The listing builds one solid part. Answer for the finished solid, in the listing's coordinates (mm). Face numbers are marked on the shaded views. A direction names the side the tool comes from. Round coordinates to 2 decimals unless told otherwise and drop trailing zeros. Order: outer loops, then holes, each group sorted by start corner. A loop starts at its lowest first (then second) coordinate and runs counter-clockwise, first axis right, second up. Notation, with made-up numbers: (7, 55.25) -> (41, 55.25) arc R19 ccw to (41, 74.25) -> close; hole circle Ø5 at (-40, -37.5). An arc over 180 degrees is marked (long way). Answer in a Markdown table with one row per item. Add a question column.
```python
from build123d import *

# Parameters (mm, degrees)
F1_DEPTH = 15.875
F2_DEPTH = 0.79375
F4_DEPTH = 0.79375
F6_DEPTH = 5.08


# Not quite as in the source:
# - a length typed as a fraction of an inch, garbled in the dataset ("3 / 203.2 mm" for 3/8 in), is restored


with BuildPart() as f1:
    # F0 (on Top) → F1 (new body)
    with BuildSketch(Plane.XY):
        with BuildLine():
            Line((-5.732164003, 16.9486273388), (-8.1134518534, 16.9486273388))
            ThreePointArc((-8.1134518534, 16.9486273388), (3.7927981466, 5.1022697967), (15.6990481466, 16.9486273388))
            Line((15.6990481466, 16.9486273388), (13.3177602962, 16.9486273388))
            ThreePointArc((13.3177602962, 16.9486273388), (3.7927981466, 7.4835197967), (-5.732164003, 16.9486273388))
        make_face()
    extrude(amount=F1_DEPTH)

    # F0 (on Top) → F2 (join)
    with BuildSketch(Plane.XY):
        with BuildLine():
            Line((13.3177602962, 16.9486273388), (-5.732164003, 16.9486273388))
            ThreePointArc((-5.732164003, 16.9486273388), (3.7927981466, 7.4835197967), (13.3177602962, 16.9486273388))
        make_face()
    extrude(amount=F2_DEPTH)

    # F3 (on face) → F4 (join)
    with BuildSketch(Plane.XY.offset(15.875)):
        with BuildLine():
            Line((13.3177602962, 16.9486273388), (-5.732164003, 16.9486273388))
            ThreePointArc((-5.732164003, 16.9486273388), (3.7927981466, 7.4236651892), (13.3177602962, 16.9486273388))
        make_face()
        with BuildLine():
            ThreePointArc((13.3177602962, 16.9486273388), (3.7927981466, 7.4236651892), (-5.732164003, 16.9486273388))
            Line((-5.732164003, 16.9486273388), (-8.1134518534, 16.9486273388))
            ThreePointArc((-8.1134518534, 16.9486273388), (3.7927981466, 5.1022697967), (15.6990481466, 16.9486273388))
            Line((15.6990481466, 16.9486273388), (13.3177602962, 16.9486273388))
        make_face()
    extrude(amount=F4_DEPTH)

    # F5 (on face) → F6 (cut)
    with BuildSketch(Plane(origin=(0, 0, 0), x_dir=(1, 0, 0), z_dir=(0, 0, -1))):
        with BuildLine():
            ThreePointArc((6.1740481466, -16.9486273388), (3.7927981466, -14.5673773388), (1.4115481466, -16.9486273388))
            Line((1.4115481466, -16.9486273388), (6.1740481466, -16.9486273388))
        make_face()
    extrude(amount=-F6_DEPTH, mode=Mode.SUBTRACT)


solid = f1.part
```
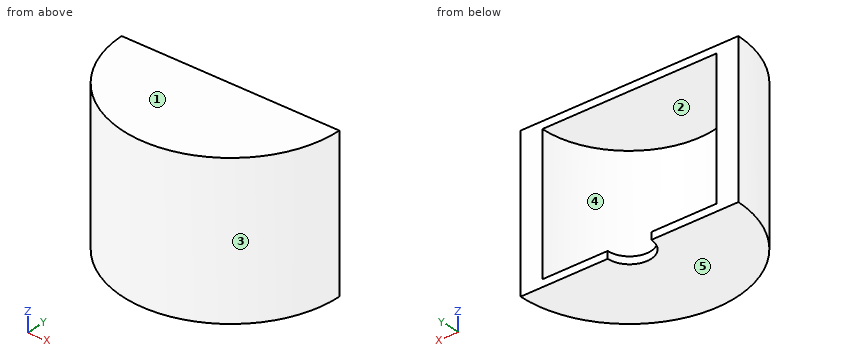
Item 1: Flat-ended cylindrical pins translate along their axes: P1, Ø2, axis at y = 7.5, z = 13.5, coming from the -X side; P2, Ø1, axis at y = 11, z = 13.5, coming from the -X side; P3, Ø3, axis at y = 10, z = 2.5, coming from the +X side. Find the tip coordinate at first contact, or state that the pin passes through.
Item 2: The part is cut by section B-B, the plane x = -1.5. Give the vertices of the cut face in (y, z) (3 decimals), and give its area (3 significant figures).
Item 3: A tool of negligible diameter and unlimited length cuts with its end or side. For the marked faces 4 and 5, from which of +Z, -Z, +X, -X, +Y, -Y can it reach the whole face along a straight path? Write none if from no direction.
Item 4: The part is cut by section D-D, the plane y = 15.75. Give the vertices of the cut face in (x, z) (3 decimals), and give its area (3 significant figures).
Item 5: The part is cut by section A-A, the plane y = 8. Give the vertices of the cut face in (x, z) (3 decimals), and give its area (3 significant figures).
Item 6: For a pull along X with two mould halves and no side action, classify the marked faces 1, 2 and 3 as released by +X, released by -X, zero draft, split by the parting line, or undercut.
Item 7: Find the intervals of material crossed by probe 1 along Z at (x, y) = (-2.25, 13.75) (3 decimals); probe 2 along X at (y, z) = (16.75, 12.5); probe 3 along X at (y, z) = (13, 3.5), in increasing order. Write a range as [from, to].
Resolved:
| question | item | result |
|---|---|---|
| 1 | P1 | x = -4.54 |
| 1 | P2 | x = -6.76 |
| 1 | P3 | x = 14.35 |
| 2 | outline | (6.343, 0) -> (16.949, 0) -> (16.949, 0.794) -> (9.089, 0.794) -> (9.089, 15.875) -> (16.949, 15.875) -> (16.949, 16.669) -> (6.343, 16.669) -> close |
| 2 | area | 58.2 mm2 |
| 3 | face 4 | +Y |
| 3 | face 5 | -Z, +X, -X, +Y, -Y |
| 4 | outline | (-8.047, 0) -> (1.735, 0) -> (1.735, 0.794) -> (-5.649, 0.794) -> (-5.649, 15.875) -> (13.234, 15.875) -> (13.234, 0.794) -> (5.85, 0.794) -> (5.85, 0) -> (15.632, 0) -> (15.632, 16.669) -> (-8.047, 16.669) -> close |
| 4 | area | 107 mm2 |
| 5 | outline | (-3.992, 0) -> (11.578, 0) -> (11.578, 16.669) -> (-3.992, 16.669) -> close; hole (0.699, 0.794) -> (6.887, 0.794) -> (6.887, 15.875) -> (0.699, 15.875) -> close |
| 5 | area | 166 mm2 |
| 6 | face 1 | zero draft |
| 6 | face 2 | undercut |
| 6 | face 3 | split by the parting line |
| 7 | probe 1 | [0, 0.794], [15.875, 16.669] |
| 7 | probe 2 | [-8.11, -5.73], [13.31, 15.7] |
| 7 | probe 3 | [-7.42, -4.85], [12.43, 15] |
